from build123d import *

# Parameters (mm, degrees)
BOSS_EXTRUDE1_DEPTH      = 11
SKETCH2_R                = 23
SKETCH2_R_2              = 14.275
BOSS_EXTRUDE2_DEPTH      = 17
BOSS_EXTRUDE3_DEPTH      = 4
SKETCH6_R                = 4
CUT_EXTRUDE1_DEPTH       = 155.964512066
BOSS_EXTRUDE4_REACH      = 172.977
BOSS_EXTRUDE4_END_RADIUS = 23
SKETCH9_R                = 8.5
SKETCH9_R_2              = 4
CUT_EXTRUDE2_REACH       = 172.977
SKETCH9_3_R              = 4
BOSS_EXTRUDE5_DEPTH      = 4
SKETCH12_R               = 14.5
SKETCH12_R_2             = 6.5
BOSS_EXTRUDE6_DEPTH      = 16.5
CUT_EXTRUDE3_DEPTH       = 171.976606706
CUT_EXTRUDE3_DEPTH_BACK  = 171.976606706
SKETCH12_2_R             = 6.5


with BuildPart() as part:
    # Sketch1 → Boss-Extrude1 (new body)
    with BuildSketch(Plane(origin=(0, 0, 0), x_dir=(1, 0, 0), z_dir=(0, 1, 0))):
        with BuildLine():
            Line((-24, -35), (24, -35))
            ThreePointArc((24, -35), (36.727922061, -29.727922061), (42, -17))
            Line((42, -17), (42, 17))
            ThreePointArc((42, 17), (36.727922061, 29.727922061), (24, 35))
            Line((24, 35), (-24, 35))
            ThreePointArc((-24, 35), (-36.727922061, 29.727922061), (-42, 17))
            Line((-42, 17), (-42, -17))
            ThreePointArc((-42, -17), (-36.727922061, -29.727922061), (-24, -35))
        make_face()
    extrude(amount=BOSS_EXTRUDE1_DEPTH)



with BuildPart() as body_2:
    # Sketch2 → Boss-Extrude2 (new, symmetric)
    with BuildSketch(Plane(origin=(0, 0, 0), x_dir=(0, 0, -1), z_dir=(1, 0, 0))):
        with Locations((0, 133)):
            Circle(SKETCH2_R)
        with Locations((0, 133)):
            Circle(SKETCH2_R_2, mode=Mode.SUBTRACT)
    extrude(amount=BOSS_EXTRUDE2_DEPTH, both=True)


with BuildPart() as part_1:
    add(part.part)

    add(body_2.part)  # Boss-Extrude3 merges body 2
    # Sketch3 → Boss-Extrude3 (add, symmetric)
    with BuildSketch(Plane(origin=(0, 0, 0), x_dir=(0, 0, -1), z_dir=(1, 0, 0))):
        with BuildLine():
            Line((-35, 11), (-22.996293992, 133.412871227))
            ThreePointArc((-22.996293992, 133.412871227), (0, 110), (22.996293992, 133.412871227))
            Line((22.996293992, 133.412871227), (35, 11))
            Line((35, 11), (-35, 11))
        make_face()
    extrude(amount=BOSS_EXTRUDE3_DEPTH, both=True)

    # Sketch6 → Cut-Extrude1 (cut, through all)
    with BuildSketch(Plane(origin=(0, 11, 0), x_dir=(1, 0, 0), z_dir=(0, 1, 0))):
        with Locations(Location((29, -23, 0), (0, 0, 270))):
            Circle(SKETCH6_R)
        with Locations(Location((29, 23, 0), (0, 0, 90))):
            Circle(SKETCH6_R)
        with Locations(Location((-29, -23, 0), (0, 0, 90))):
            Circle(SKETCH6_R)
        with Locations(Location((-29, 23, 0), (0, 0, 270))):
            Circle(SKETCH6_R)
    extrude(amount=-CUT_EXTRUDE1_DEPTH, mode=Mode.SUBTRACT)

    # Boss-Extrude4: up to this cylinder (the profile starts outside it)
    boss_extrude4_end = Plane(origin=(0, 133, 0), z_dir=(-1, 0, 0)) * Cylinder(BOSS_EXTRUDE4_END_RADIUS, 392.954, mode=Mode.PRIVATE)
    # Sketch9 → Boss-Extrude4 (add, up to the surface)
    with BuildSketch(Plane(origin=(0, 162, 0), x_dir=(-1, 0, 0), z_dir=(0, -1, 0)), mode=Mode.PRIVATE) as boss_extrude4_sk1:
        with Locations(Location((0, 0, 0), (0, 0, 270))):
            Circle(SKETCH9_R)
        with Locations(Location((0, 0, 0), (0, 0, 270))):
            Circle(SKETCH9_R_2, mode=Mode.SUBTRACT)
    boss_extrude4_tool1 = extrude(boss_extrude4_sk1.sketch, amount=BOSS_EXTRUDE4_REACH, mode=Mode.PRIVATE) - boss_extrude4_end
    add(boss_extrude4_tool1.solids().sort_by_distance((0, 162, -8.259584))[0])

    # Sketch9_3 → Cut-Extrude2 (cut, up to next)
    with BuildSketch(Plane(origin=(0, 162, 0), x_dir=(-1, 0, 0), z_dir=(0, -1, 0)), mode=Mode.PRIVATE) as cut_extrude2_sk1:
        with Locations(Location((0, 0, 0), (0, 0, 270))):
            Circle(SKETCH9_3_R)
    cut_extrude2_tool1 = extrude(cut_extrude2_sk1.sketch, amount=CUT_EXTRUDE2_REACH, mode=Mode.PRIVATE) & part_1.part
    add(cut_extrude2_tool1.solids().sort_by_distance((0, 162, 0))[0], mode=Mode.SUBTRACT)

    # Sketch10 → Boss-Extrude5 (add, symmetric)
    with BuildSketch(Plane.XY):
        with BuildLine():
            Line((14, 113), (14, 42.749015733))
            ThreePointArc((14, 42.749015733), (22, 21.583005244), (42, 11))
            Line((42, 11), (4, 11))
            Line((4, 11), (4, 113))
            Line((4, 113), (14, 113))
        make_face()
    boss_extrude5 = extrude(amount=BOSS_EXTRUDE5_DEPTH, both=True)

    # Mirror1: Boss-Extrude5 across plane
    add(boss_extrude5.mirror(Plane(origin=(0, 0, 0), x_dir=(0, 0, 1), z_dir=(1, 0, 0))))

    # Sketch12 → Boss-Extrude6 (add, symmetric)
    with BuildSketch(Plane(origin=(0, 0, 0), x_dir=(0, 0, -1), z_dir=(1, 0, 0))):
        with Locations(Location((-14, 53.219049893, 0), (0, 0, 313.602818973))):
            Circle(SKETCH12_R)
        with Locations((-14, 53.219049893)):
            Circle(SKETCH12_R_2, mode=Mode.SUBTRACT)
    extrude(amount=BOSS_EXTRUDE6_DEPTH, both=True)

    # Sketch12_2 → Cut-Extrude3 (cut, two sides: drawn at the far end of the back side and taken through both)
    with BuildSketch(Plane(origin=(0, 0, 0), x_dir=(0, 0, -1), z_dir=(1, 0, 0)).offset(-CUT_EXTRUDE3_DEPTH_BACK)):
        with Locations((-14, 53.219049893)):
            Circle(SKETCH12_2_R)
    extrude(amount=CUT_EXTRUDE3_DEPTH + CUT_EXTRUDE3_DEPTH_BACK, mode=Mode.SUBTRACT)


solid = part_1.part
Input: part model. Units: mm. Frame: model coordinates. A direction names the side the tool comes from. Give positions to 0.01 mm unless a question says otherwise; leave off trailing zeros. Order: outer loops, then holes, each group sorted by start corner. A loop starts at its lowest first (then second) coordinate and runs counter-clockwise, first axis right, second up.
Q1. Section D-D on y = 103. Output: boundary loops of the cut face in (x, z), and give its area (3 significant figures).
Checked values:
outline: (-14, -4) - (-4, -4) - (-4, -25.98) - (4, -25.98) - (4, -4) - (14, -4) - (14, 4) - (4, 4) - (4, 25.98) - (-4, 25.98) - (-4, 4) - (-14, 4) - close
area: 576 mm2
Q2. Ray query, probe 1 along X at (y, z) = (159.5, 0); probe 2 along Y at (x, z) = (-9.5, -18); probe 3 along X at (y, z) = (3, 23). Return the intervals inside material, ascending.
Checked values:
probe 1: x = -8.5 to -4, 4 to 8.5
probe 2: y = 0 to 11, 118.68 to 147.32
probe 3: x = -40.97 to -33, -25 to 25, 33 to 40.97
Q3. Contact query for flat-ended pins moving along their axis: pin 1 Ø8 at (x, y) = (-7, 77.5) entering from +Z; pin 2 Ø10 at (x, z) = (10.5, -19) entering from -Y; pin 3 Ø15.5 at (y, z) = (98.5, -17) entering from +X; pin 4 Ø25 at (x, z) = (-22, 14) entering from +Y. Output: stop coordinate, or through.
Checked values:
pin 1: stops at z = 28.74
pin 2: stops at y = 0
pin 3: stops at x = 4
pin 4: stops at y = 155.86
Q4. Draft query along Z for faces 4 (the cylindrical face through (-36.587, 5.423, -29.867)), 5 (the flat face through (-16.5, 46.7, 16.4)), 6 (the cylindrical face through (-10.162, 55.467, 28.325)), 7 (the cylindrical face through (32.966, 5.577, 22.479)). Return one class per face: +Z half, -Z half, draft (parallel to the pull), parting line (faces both ways), or undercut.
Checked values:
face 4: -Z half
face 5: draft
face 6: undercut
face 7: undercut
Q5. Set-up query: faces 1 (the flat face through (0, 5, -35)), 2 (the flat face through (23, 11, -20)), 3 (the flat face through (-17, 123, 11)). Return all of +Z, -Z, +X, -X, +Y, -Y with unobstructed straight access to the full face (end or side cutting, diameter ignored); none if empty.
Checked values:
face 1: -Z, +X, -X, +Y, -Y
face 2: -Z, +X
face 3: +Z, -Z, -X, +Y
Q6. Section A-A on y = 136. Output: boundary loops of the cut face in (x, z).
Checked values:
outline: (-17, -22.8) - (17, -22.8) - (17, -13.96) - (-17, -13.96) - close; (-17, 13.96) - (17, 13.96) - (17, 22.8) - (-17, 22.8) - close
Q7. Section B-B on x = -29. Output: boundary loops of the cut face in (y, z), and give its area (3 significant figures).
Checked values:
outline: (0, -34.29) - (11, -34.29) - (11, -27) - (0, -27) - close; (0, -19) - (11, -19) - (11, -4) - (15.64, -4) - (15.64, 4) - (11, 4) - (11, 19) - (0, 19) - close; (0, 27) - (11, 27) - (11, 34.29) - (0, 34.29) - close
area: 616 mm2
Q8. Section C-C on x = 6.5. State how many separate pieces and enclosed holes the cut face has, and give its area (3 significant figures).
Checked values:
separate pieces: 1
enclosed holes: 2
area: 3,120 mm2
